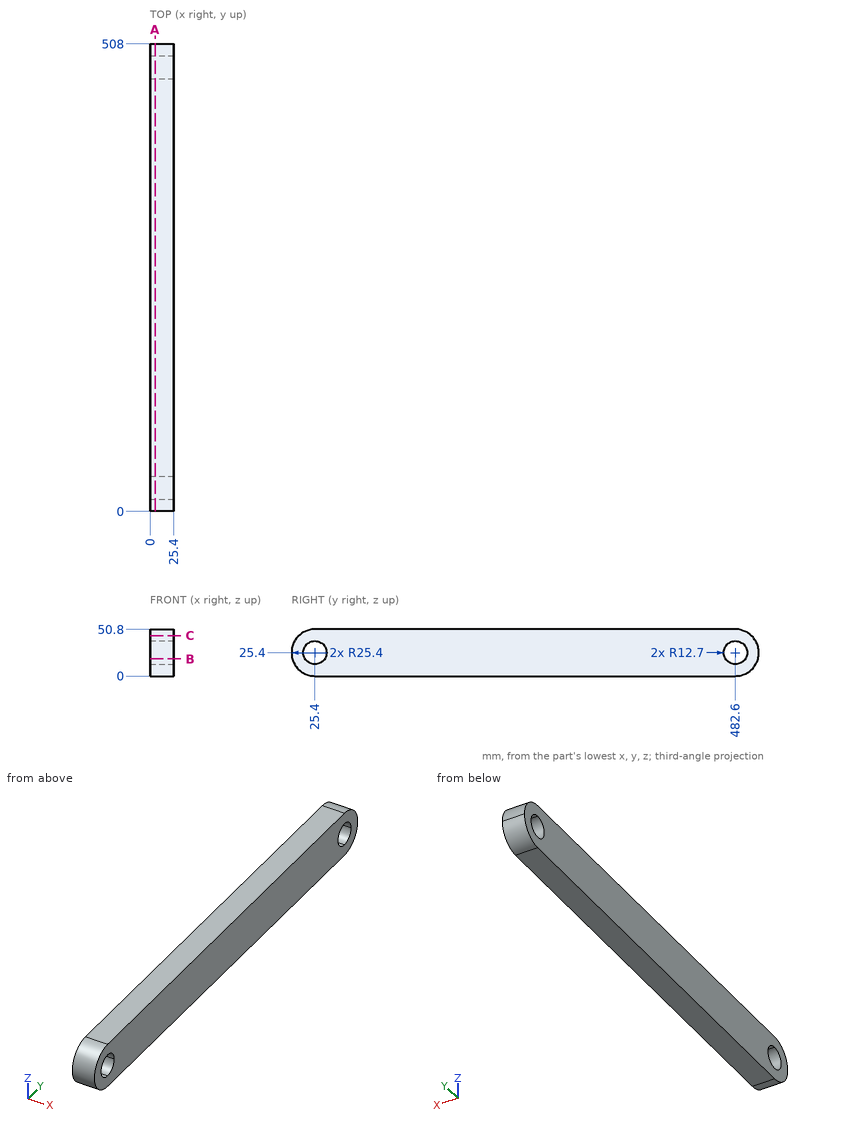
The drawing under review shows one solid part. Ordinate dimensions are in mm from its lowest x, y, z. Give positions to 0.01 mm unless a question says otherwise; leave off trailing zeros. Write each loop counter-clockwise with the first axis right and the second up, starting at its lowest first coordinate (ties: lowest second). Pieces come first, ordered by that corner, then holes. Notation, with made-up numbers: (1, 19) -> (12, 19) arc R31 cw to (12, 49) -> close; hole circle Ø4 at (-30.5, -33). An arc over 180 degrees is marked (long way). Put each result on its own line as item: value.
(1) To check wall thickness, follow probe 1 along Y at (x, z) = (20.25, 24.5); probe 2 along Y at (x, z) = (24.5, 14.5); probe 3 along Z at (x, y) = (5.75, 480). State the ranges of each line that lie inside material, in increasing order. Write a range as from..to.
Results are:
probe 1: 0.02..12.73, 38.07..469.93, 495.27..507.98
probe 2: 2.46..18.88, 31.92..476.08, 489.12..505.54
probe 3: 0..12.97, 37.83..50.8
(2) We need section B-B, the plane z = 18.5. Give the boundary of the cut face in (x, y).
Results are:
outline: (0, 0.96) -> (25.4, 0.96) -> (25.4, 14.74) -> (0, 14.74) -> close; (0, 36.06) -> (25.4, 36.06) -> (25.4, 471.94) -> (0, 471.94) -> close; (0, 493.26) -> (25.4, 493.26) -> (25.4, 507.04) -> (0, 507.04) -> close
(3) For pin 1 Ø1.5 at (x, z) = (20, 45) entering from +Y; pin 2 Ø5 at (x, z) = (6.5, 40.5) entering from +Y; pin 3 Ø4 at (x, z) = (20, 12) entering from +Y, all flat-tipped, find the tip position at first contact; note any pin that passes through.
Results are:
pin 1: y = 499.62
pin 2: y = 504.65
pin 3: y = 505.3
(4) We need section A-A, the plane x = 5.5. Give the boundary of the cut face in (y, z), and give its area (3 significant figures).
Results are:
outline: (25.4, 0) -> (482.6, 0) arc R25.4 ccw to (482.6, 50.8) -> (25.4, 50.8) arc R25.4 ccw to start; hole circle Ø25.4 at (25.4, 25.4); hole circle Ø25.4 at (482.6, 25.4)
area: 24,200 mm²
(5) We need section C-C, the plane z = 44. Give the boundary of the cut face in (x, y), and give its area (3 significant figures).
Results are:
outline: (0, 8.1) -> (25.4, 8.1) -> (25.4, 499.9) -> (0, 499.9) -> close
area: 12,500 mm²
